Geometry: final body of the model. Coordinates: model frame, mm. Face numbers are marked on the shaded views. A direction names the side the tool comes from. Give positions to 0.01 mm unless a question says otherwise; leave off trailing zeros. Write each loop counter-clockwise with the first axis right and the second up, starting at its lowest first coordinate (ties: lowest second). Pieces come first, ordered by that corner, then holes.
```python
from build123d import *

# Parameters (mm, degrees)
BOSS_EXTRUDE1_DEPTH   = 88.9
SKETCH2_W             = 88.9
SKETCH2_H             = 50.8
BOSS_EXTRUDE2_DEPTH   = 3.175
FILLET2_DEPTH         = 25.4
FILLET2_START         = 63.5
FILLET2_2_DEPTH       = 25.4
FILLET2_START_2       = 25.4
FILLET2_3_DEPTH       = 38.1
FILLET2_4_DEPTH       = 38.1
FILLET2_START_3       = -25.4
FILLET2_5_OUTLINE_W   = 3.175
FILLET2_5_OUTLINE_H   = 50.8
FILLET2_5_DEPTH       = 139.7
FILLET2_START_4       = -10.570754214
FILLET2_6_OUTLINE_R   = 3.302
FILLET2_6_OUTLINE_R_2 = 3.175
FILLET2_6_DEPTH       = 3.175


with BuildPart() as part:
    # Sketch1 → Boss-Extrude1 (new body)
    with BuildSketch(Plane(origin=(0, 0, 0), x_dir=(0, 0, -1), z_dir=(1, 0, 0))):
        Polygon((27.601330486, -7.395754214), (-23.198669514, -7.395754214), (-27.601330486, 7.395754214), align=None)
    extrude(amount=BOSS_EXTRUDE1_DEPTH)

    # Sketch2 → Boss-Extrude2 (add)
    with BuildSketch(Plane.XZ.offset(7.395754214)):
        with Locations((44.45, -2.201330486)):
            Rectangle(SKETCH2_W, SKETCH2_H)
    extrude(amount=BOSS_EXTRUDE2_DEPTH)

    # Fillet2: read off the stored shape, not the designer's step
    # Fillet2 outline → Fillet2 (cut)
    with BuildSketch(Plane.YZ):
        Polygon((-7.395754214, 23.198669514), (-7.395754214, -27.601330486), (7.395754214, 27.601330486), align=None)
    extrude(amount=FILLET2_DEPTH, mode=Mode.SUBTRACT)

    # Fillet2 2 outline → Fillet2 2 (cut)
    with BuildSketch(Plane.YZ.offset(FILLET2_START)):
        Polygon((-7.395754214, 23.198669514), (-7.395754214, -27.601330486), (7.395754214, 27.601330486), align=None)
    extrude(amount=FILLET2_2_DEPTH, mode=Mode.SUBTRACT)

    # Fillet2 3 outline → Fillet2 3 (cut)
    with BuildSketch(Plane.YZ.offset(FILLET2_START_2)):
        with BuildLine():
            Line((7.395754214, 27.601330486), (-7.00664086, 23.314488275))
            ThreePointArc((-7.00664086, 23.314488275), (-5.264031089, 23.20711322), (-4.002401192, 22.000254398))
            ThreePointArc((-4.002401192, 22.000254398), (-0.667927102, 17.789753466), (4.108752341, 15.334072492))
            Line((4.108752341, 15.334072492), (7.395754214, 27.601330486))
        make_face()
    extrude(amount=FILLET2_3_DEPTH, mode=Mode.SUBTRACT)

    # Fillet2 4 outline → Fillet2 4 (add)
    with BuildSketch(Plane.YZ.offset(FILLET2_START_2)):
        with BuildLine():
            Line((4.108752341, 15.334072492), (-7.395754214, -27.601330486))
            Line((-7.395754214, -27.601330486), (-7.730151558, -27.601330486))
            ThreePointArc((-7.730151558, -27.601330486), (-7.39861503, -27.623060538), (-7.072751183, -27.687878887))
            Line((-7.072751183, -27.687878887), (4.87150378, -30.888332359))
            Line((4.87150378, -30.888332359), (16.376010335, 12.04707062))
            Line((16.376010335, 12.04707062), (4.108752341, 15.334072492))
        make_face()
    extrude(amount=FILLET2_4_DEPTH)

    # Fillet2 5 outline → Fillet2 5 (add)
    with BuildSketch(Plane.YZ.offset(FILLET2_START_3)):
        with Locations((-8.983254214, -2.201330486)):
            Rectangle(FILLET2_5_OUTLINE_W, FILLET2_5_OUTLINE_H)
    extrude(amount=FILLET2_5_DEPTH)

    # Fillet2 6 outline → Fillet2 6 (cut)
    with BuildSketch(Plane(origin=(0, 0, 0), x_dir=(1, 0, 0), z_dir=(0, 1, 0)).offset(FILLET2_START_4)):
        with Locations((101.6, -10.498669514)):
            Circle(FILLET2_6_OUTLINE_R)
        with Locations((101.6, 14.901330486)):
            Circle(FILLET2_6_OUTLINE_R)
        with Locations((-12.7, -10.498669514)):
            Circle(FILLET2_6_OUTLINE_R_2)
        with Locations((-12.7, 14.901330486)):
            Circle(FILLET2_6_OUTLINE_R_2)
    extrude(amount=FILLET2_6_DEPTH, mode=Mode.SUBTRACT)


solid = part.part
```
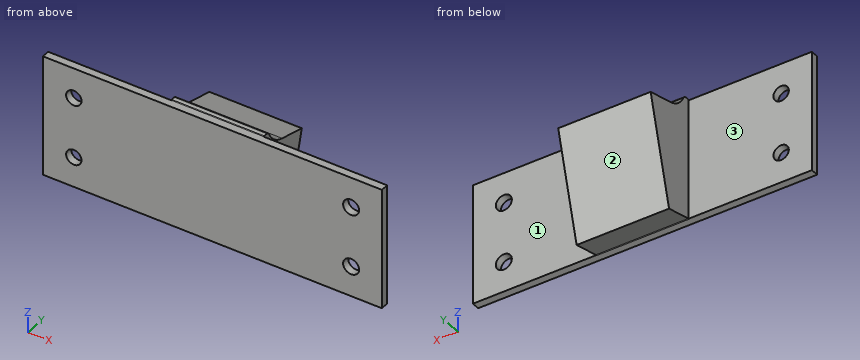
Item 1: Section B-B, the plane x = 42. Return the cut outline in (y, z).
Found:
outline: (-10.57, -27.6) - (-7.73, -27.6) arc R2.54 cw to (-7.07, -27.69) - (4.87, -30.89) - (16.38, 12.05) - (4.11, 15.33) arc R12.7 cw to (-4, 22) arc R2.54 ccw to (-7.01, 23.31) - (-7.4, 23.2) - (-10.57, 23.2) - close
Item 2: Reachability of the marked faces 1, 2 and 3 from +Z, -Z, +X, -X, +Y, -Y: full face, straight path, thin tool, end or side. Return the list, or none.
Found:
face 1: +Z, -Z, +X, +Y
face 2: -Z, +X, -X, +Y
face 3: +Z, -Z, -X, +Y
Item 3: Pin query (flat end, axial travel): pin 1 Ø6 at (x, z) = (101.6, 10.5) entering from -Y; pin 2 Ø1.5 at (y, z) = (0.5, -5) entering from +X; pin 3 Ø15 at (x, z) = (-7.5, 7) entering from +Y; pin 4 Ø7 at (y, z) = (10, 2.5) entering from -X. Return the tip coordinate at first contact, or that it passes through.
Found:
pin 1: passes through
pin 2: stops at x = 63.5
pin 3: stops at y = -7.4
pin 4: stops at x = 25.4
Item 4: Section D-D, the plane x = -12.7. Return the cut outline in (y, z), plus the area to 3 significant figures.
Found:
outline: (-10.57, -27.6) - (-7.4, -27.6) - (-7.4, -18.08) - (-10.57, -18.08) - close; (-10.57, -11.73) - (-7.4, -11.73) - (-7.4, 7.32) - (-10.57, 7.32) - close; (-10.57, 13.67) - (-7.4, 13.67) - (-7.4, 23.2) - (-10.57, 23.2) - close
area: 121 mm2
Item 5: Line query: L1, parallel to Z at x = -12.7, y = -8.6; L2, parallel to Z at x = 101.6, y = -9.5; L3, parallel to X at y = -5.75, z = -23.5. Output: solid intervals per line, ascending.
Found:
L1: z = -27.6 to -18.08, -11.73 to 7.32, 13.67 to 23.2
L2: z = -27.6 to -18.2, -11.6 to 7.2, 13.8 to 23.2
L3: x = 25.4 to 63.5
Item 6: Section A-A, the plane x = 101.6. Return the cut outline in (y, z), plus the area to 3 significant figures.
Found:
outline: (-10.57, -27.6) - (-7.4, -27.6) - (-7.4, -18.2) - (-10.57, -18.2) - close; (-10.57, -11.6) - (-7.4, -11.6) - (-7.4, 7.2) - (-10.57, 7.2) - close; (-10.57, 13.8) - (-7.4, 13.8) - (-7.4, 23.2) - (-10.57, 23.2) - close
area: 119 mm2
Item 7: Section C-C, the plane z = -10. Return the cut outline in (x, y).
Found:
outline: (-25.4, -10.57) - (114.3, -10.57) - (114.3, -7.4) - (63.5, -7.4) - (63.5, 10.47) - (25.4, 10.47) - (25.4, -7.4) - (-25.4, -7.4) - close
